Autodesk Inventor part; units mm, degrees
ref_plane "YZ Plane" through (0, 0, 0) normal (1, 0, 0) x (0, 1, 0)
ref_plane "XZ Plane" through (0, 0, 0) normal (0, 1, 0) x (-1, 0, 0)
ref_plane "XY Plane" through (0, 0, 0) normal (0, 0, 1) x (1, 0, 0)
sketch "Boceto2" plane through (0, 0, 0) normal (0, 1, 0) x (-1, 0, 0)
  arc A0 (5, 0) -> (-5, 0) centre (0, 0) ccw
  arc A1 (1.2, 2.1932) -> (1.2, -2.1932) centre (0, 0) ccw
  line L0 (1.2, 2.1932) -> (1.2, -2.1932)
  line L1 (0, 0) -> (0, -180) construction
  circle A2 centre (0, -180) radius 8.75
  arc A3 (-6.8254, -171.6948) -> (6.8254, -171.6948) centre (0, -180) ccw
  line L2 (5, -11.1803) -> (5, -167.8319)
  line L3 (-5, -11.1803) -> (-5, -167.8319)
  arc A4 (-6.8254, -171.6948) -> (-5, -167.8319) centre (-10, -167.8319) ccw
  arc A5 (5, -167.8319) -> (6.8254, -171.6948) centre (10, -167.8319) ccw
  arc A6 (6.6667, -7.4536) -> (-6.6667, -7.4536) centre (0, 0) ccw
  arc A7 (6.6667, -7.4536) -> (5, -11.1803) centre (10, -11.1803) ccw
  arc A8 (-5, -11.1803) -> (-6.6667, -7.4536) centre (-10, -11.1803) ccw
  point P0 (-5, -170.4836)
  point P1 (5, -170.4836)
  point P2 (5, -8.6603)
  point P3 (-5, -8.6603)
  dimension "d13" = 10
  dimension "d14" = 5
  dimension "d15" = 1.2
  dimension "d16" = 180
  dimension "d17" = 17.5
  dimension "d18" = 2
  dimension "d19" = 5
  dimension "d27" = 20
  dimension "d28" = 5
  dimension "d29" = 5
extrude "Extrusión2" add sketch "Boceto2" along normal blind 10
sketch "Boceto3" plane through (0, 10, 0) normal (0, 1, 0) x (1, 0, 0)
  circle A0 centre (0, 0) radius 4
  line L0 (-3, -2.6458) -> (-3, 2.6458)
  line L1 (-3, -2.6458) -> (4.3142, -2.6458) construction
  dimension "d22" = 8
  dimension "d25" = 90
  dimension "d26" = 3
extrude "Extrusión3" cut sketch "Boceto3" against normal blind 10 contours A0 L0 picked at (0.3596, 0.8073)
properties part number "eslabon2"
Could you check a few things on this model? Use its own coordinates, in mm. A direction names the side the tool comes from. Round coordinates to 2 decimals unless told otherwise and drop trailing zeros. Order: outer loops, then holes, each group sorted by start corner. A loop starts at its lowest first (then second) coordinate and runs counter-clockwise, first axis right, second up. Notation, with made-up numbers: M 79,-15 L 100,-15 A21 cw 100,15 Z; hole C 41.25,89 d9. An arc over 180 degrees is marked long. One line per item, written item: value.
(1) I need wall thicknesses on line 1 along X through (y, z) = (3.75, 0); line 2 along Z through (x, y) = (6.5, 5); line 3 along Z through (x, y) = (6.25, 6.75). Which ranges of each line are inside material? Lowest first, please. Write a range as from..to.
Ans:
line 1: x = -10..-3, 4..10
line 2: z = -188.56..-185.86, -174.14..-171.4, -7.61..7.6
line 3: z = -188.75..-186.12, -173.88..-171.14, -7.87..7.81
(2) Imagine slicing it at D-D (z = 0). Write out the boundary of the cut face in (x, y).
Ans:
outline: M -10,0 L -3,0 L -3,10 L -10,10 Z; M 4,0 L 10,0 L 10,10 L 4,10 Z
(3) Imagine slicing it at B-B (x = -0.5). Write out the boundary of the cut face in (y, z), and give its area (3 significant figures).
Ans:
outline: M 0,-190.74 L 10,-190.74 L 10,-188.74 L 0,-188.74 Z; M 0,-171.26 L 10,-171.26 L 10,-3.97 L 0,-3.97 Z; M 0,3.97 L 10,3.97 L 10,9.99 L 0,9.99 Z
area: 1,750 mm^2
(4) Which directions (+Z, -Z, +X, -X, +Y, -Y) give clear straight access to the entire face, cutting with the end or side of a thin tool? Please do faces 1 (the flat face through (5, 5, -88)), 2 (the cylindrical face through (-5.493, 4.93, -169.996)), 3 (the flat face through (-3, 5, 0)).
Ans:
face 1: +X, +Y, -Y
face 2: -X, +Y, -Y
face 3: +Y, -Y
(5) I'm going to push flat-ended pins straight in: P1, Ø1.5, axis at y = 3, z = -71.5, coming from the -X side; P2, Ø2.5, axis at y = 3, z = 1, coming from the +X side; P3, Ø1, axis at x = 6.5, y = 2, coming from the -Z side. Where does each tip first touch, or does it pass through?
Ans:
P1: stops at x = -5
P2: stops at x = 10
P3: stops at z = -188.92
(6) Imagine slicing it at A-A (z = -180). Write out the boundary of the cut face in (x, y), and give its area (3 significant figures).
Ans:
outline: M -10.75,0 L -8.75,0 L -8.75,10 L -10.75,10 Z; M 8.75,0 L 10.75,0 L 10.75,10 L 8.75,10 Z
area: 40.0 mm^2
(7) Imagine slicing it at C-C (y = 4.5). Write out the boundary of the cut face in (x, z), and give its area (3 significant figures).
Ans:
outline: M -6.83,-171.69 A10.75 ccw long 6.83,-171.69 A5 cw 5,-167.83 L 5,-11.18 A5 cw 6.67,-7.45 A10 ccw long -6.67,-7.45 A5 cw -5,-11.18 L -5,-167.83 A5 cw Z; hole C 0,-180 d17.5; hole M -3,-2.65 A4 ccw long -3,2.65 Z
area: 1,990 mm^2
(8) If we mould it in two halves opening along Z, with no side actions, what happens to faces 4 (the flat face through (0, 10, -89)), 5 (the flat face through (-5, 5, -88))? For each: released by +Z, released by -Z, zero draft, split by the parting line, or undercut.
Ans:
face 4: zero draft
face 5: undercut
